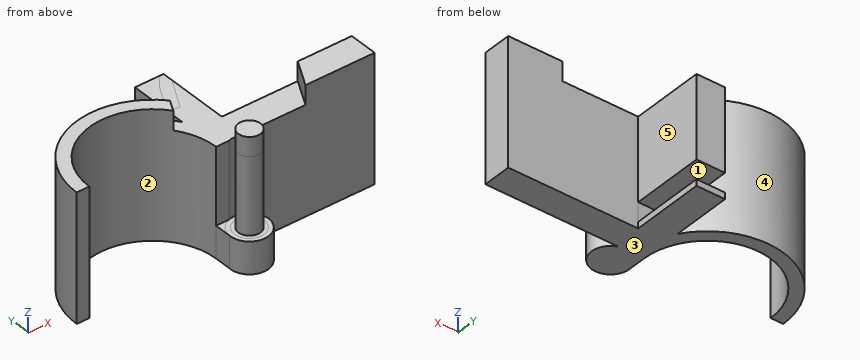
from build123d import *

# Parameters (mm, degrees)
BOSS_EXTRUDE1_DEPTH = 20
SKETCH7_R           = 1.75
BOSS_EXTRUDE5_DEPTH = 20
BOSS_EXTRUDE6_DEPTH = 5
SKETCH8_W           = 25
SKETCH8_H           = 20
BOSS_EXTRUDE7_DEPTH = 4.5
SKETCH9_W           = 4.5
SKETCH9_H           = 20
BOSS_EXTRUDE8_DEPTH = 16
SKETCH10_R          = 1.75
CUT_EXTRUDE1_DEPTH  = 3
SKETCH12_R          = 1.75
BOSS_EXTRUDE9_DEPTH = 3
SKETCH14_R          = 3
SKETCH14_R_2        = 2.333892431
CUT_EXTRUDE3_DEPTH  = 16
CUT_EXTRUDE4_DEPTH  = 3
SKETCH16_W          = 3
SKETCH16_H          = 11.5
CUT_EXTRUDE5_DEPTH  = 5


with BuildPart() as part:
    # Sketch1 → Boss-Extrude1 (new body)
    with BuildSketch(Plane.XY):
        with BuildLine():
            Line((-12, 0), (-10, 0))
            ThreePointArc((-10, 0), (0, 10), (10, 0))
            Line((10, 0), (12, 0))
            ThreePointArc((12, 0), (11.984990613, 0.6), (11.94, 1.198499061))
            ThreePointArc((11.94, 1.198499061), (11.893303563, 1.596662255), (11.833333333, 1.993043457))
            ThreePointArc((11.833333333, 1.993043457), (-1, 11.958260743), (-12, 0))
        make_face()
    extrude(amount=BOSS_EXTRUDE1_DEPTH)



with BuildPart() as body_2:
    # Sketch7 → Boss-Extrude5 (new body)
    with BuildSketch(Plane(origin=(0, 0, 0), x_dir=(-1, 0, 0), z_dir=(0, 0, -1))):
        with Locations((-12.991756156, -2.831328262)):
            Circle(SKETCH7_R)
    extrude(amount=-BOSS_EXTRUDE5_DEPTH)

    # Sketch5 → Boss-Extrude6 (add)
    with BuildSketch(Plane(origin=(0, 0, 0), x_dir=(-1, 0, 0), z_dir=(0, 0, -1))):
        with BuildLine():
            Line((-10, 0), (-10, -2.609078175))
            ThreePointArc((-10, -2.609078175), (-15.372704459, -4.656454335), (-12, 0))
            Line((-12, 0), (-10, 0))
        make_face()
    extrude(amount=-BOSS_EXTRUDE6_DEPTH)


with BuildPart() as part_1:
    add(part.part)

    add(body_2.part)  # Boss-Extrude7 merges body 2
    # Sketch8 → Boss-Extrude7 (add)
    with BuildSketch(Plane(origin=(0, 0, 0), x_dir=(1, 0, 0), z_dir=(0, 1, 0))):
        with Locations((22.5, -10)):
            Rectangle(SKETCH8_W, SKETCH8_H)
    extrude(amount=BOSS_EXTRUDE7_DEPTH)

    # Sketch9 → Boss-Extrude8 (add)
    with BuildSketch(Plane.XZ):
        with Locations((12.25, 10)):
            Rectangle(SKETCH9_W, SKETCH9_H)
    extrude(amount=-BOSS_EXTRUDE8_DEPTH)

    # Sketch10 → Cut-Extrude1 (cut)
    with BuildSketch(Plane.XY.offset(20)):
        with BuildLine():
            Line((10, 0), (24.09729333, 0))
            Line((24.09729333, 0), (26.472308955, 4.5))
            Line((26.472308955, 4.5), (14.5, 4.5))
            Line((14.5, 4.5), (14.5, 16))
            Line((14.5, 16), (14.022774425, 16))
            ThreePointArc((14.022774425, 16), (12.880514361, 14.832204973), (11.982740375, 13.467468681))
            Line((11.982740375, 13.467468681), (10, 9.710722159))
            Line((10, 9.710722159), (10, 6.633249581))
            ThreePointArc((10, 6.633249581), (9.540752339, 7.278327061), (9.039960442, 7.891711805))
            Line((9.039960442, 7.891711805), (8.02434549, 5.967401399))
            ThreePointArc((8.02434549, 5.967401399), (9.493246413, 3.142971929), (10, 0))
        make_face()
        with Locations(Location((12.991756156, -2.831328262, 0), (0, 0, 180))):
            Circle(SKETCH10_R)
    extrude(amount=-CUT_EXTRUDE1_DEPTH, mode=Mode.SUBTRACT)

    # Sketch12 → Boss-Extrude9 (add)
    with BuildSketch(Plane.XY.offset(17)):
        with Locations(Location((12.991756156, -2.831328262, 0), (0, 0, 180))):
            Circle(SKETCH12_R)
    extrude(amount=BOSS_EXTRUDE9_DEPTH)

    # Sketch14 → Cut-Extrude3 (cut)
    with BuildSketch(Plane.XY.offset(5)):
        with Locations((12.991756156, -2.831328262)):
            Circle(SKETCH14_R)
        with Locations((12.991756156, -2.831328262)):
            Circle(SKETCH14_R_2, mode=Mode.SUBTRACT)
    extrude(amount=CUT_EXTRUDE3_DEPTH, mode=Mode.SUBTRACT)

    # Sketch15 → Cut-Extrude4 (cut)
    with BuildSketch(Plane.XY.offset(20)):
        Polygon((9.332134569, 17.011722294), (15.835730862, 16.761583975), (11.722345172, 9.285227553), (9.050959886, 9.701180523), align=None)
    extrude(amount=-CUT_EXTRUDE4_DEPTH, mode=Mode.SUBTRACT)

    # Sketch16 → Cut-Extrude5 (cut)
    with BuildSketch(Plane(origin=(14.5, 0, 0), x_dir=(0, 0, -1), z_dir=(1, 0, 0))):
        with Locations((-2.5, 10.25)):
            Rectangle(SKETCH16_W, SKETCH16_H)
    extrude(amount=-CUT_EXTRUDE5_DEPTH, mode=Mode.SUBTRACT)


solid = part_1.part
The listing builds one solid part. Answer for the finished solid, in the listing's coordinates (mm). Face numbers are marked on the shaded views. A direction names the side the tool comes from. Give positions to 0.01 mm unless a question says otherwise; leave off trailing zeros. Loops run counter-clockwise (first coordinate to the right, second up) from the corner with the lowest first, then second, coordinate; pieces in that order, holes last.
Item 1: A tool of negligible diameter and unlimited length cuts with its end or side. For the marked faces 1 and 2, from which of +Z, -Z, +X, -X, +Y, -Y can it reach the whole face along a straight path? Write none if from no direction.
Derived:
face 1: +X, +Y
face 2: +Z, -Z, -Y
Item 2: Determine the mould class of the marked faces 3, 4 and 5 for opening direction X: +X half, -X half, draft (parallel to the pull), parting line (faces both ways), or undercut.
Derived:
face 3: draft
face 4: undercut
face 5: +X half
Item 3: A cutting plane is placed at A-A (y = 12.75). Give the vertices of the cut face in (x, z), then the cut area to 3 significant figures.
Derived:
outline: (10, 0) - (14.5, 0) - (14.5, 1) - (10, 1) - close; (10, 4) - (14.5, 4) - (14.5, 17) - (10, 17) - close
area: 63.0 mm2
Item 4: A cutting plane is placed at C-C (z = 18). Give the vertices of the cut face in (x, y).
Derived:
outline: (-12, 0) - (-10, 0) arc R10 cw to (8.02, 5.97) - (9.04, 7.89) arc R12 ccw to start; circle Ø3.5 at (12.99, -2.83); (24.1, 0) - (35, 0) - (35, 4.5) - (26.47, 4.5) - close
Item 5: Each of these flat-tipped pins is pushed along its axis until it touches: pin 1 Ø11.5 at (x, y) = (21, 8) entering from +Z; pin 2 Ø2 at (x, z) = (29, 12.5) entering from -Y; pin 3 Ø1 at (x, y) = (11, -1.5) entering from +Z; pin 4 Ø3 at (x, y) = (21, 1) entering from -Z. Where does it stop, or does it pass through?
Derived:
pin 1: stops at z = 17
pin 2: stops at y = 0
pin 3: stops at z = 5
pin 4: stops at z = 0
Item 6: Find the intervals of material crossed by line 1 along X through (y, z) = (7, 10.5); line 2 along Z through (x, y) = (14, -0.5); line 3 along X through (y, z) = (5.25, 5.5), in increasing order.
Derived:
line 1: x = -9.75 to -7.14, 7.14 to 9.75, 10 to 14.5
line 2: z = 0 to 5
line 3: x = -10.79 to -8.51, 8.51 to 14.5
Item 7: A cutting plane is placed at B-B (z = 11.25). Give the vertices of the cut face in (x, y), then the cut area to 3 significant figures.
Derived:
outline: (-12, 0) - (-10, 0) arc R10 cw to (10, 0) - (12, 0) arc R3 cw to (13.98, 0) - (35, 0) - (35, 4.5) - (14.5, 4.5) - (14.5, 16) - (10, 16) - (10, 6.63) arc R12 ccw to start; circle Ø3.5 at (12.99, -2.83)
area: 234 mm2
Item 8: A cutting plane is placed at D-D (x = 19.5). Give the vertices of the cut face in (y, z).
Derived:
outline: (0, 0) - (4.5, 0) - (4.5, 17) - (0, 17) - close
